```python
from build123d import *

# Parameters (mm, degrees)
F0_R     = 7
F0_R_2   = 2.25
F1_DEPTH = 2
F2_SIZE  = 1.99999


# Not quite as in the source:
# - a fillet or chamfer is up to 0.001 mm smaller than in the source, because OpenCascade refuses the exact size


with BuildPart() as f1:
    # F0 (on Top) → F1 (new body)
    with BuildSketch(Plane.XY):
        with BuildLine():
            ThreePointArc((11.7645575334, 8.4761539653), (10.9717281133, 9.333063578), (10.2530483272, 10.2530483272))
            ThreePointArc((10.2530483272, 10.2530483272), (0, 14.5), (-10.2530483272, 10.2530483272))
            ThreePointArc((-10.2530483272, 10.2530483272), (-10.9717281133, 9.333063578), (-11.7645575334, 8.4761539653))
            ThreePointArc((-11.7645575334, 8.4761539653), (-14.5, 0), (-11.7645575334, -8.4761539653))
            ThreePointArc((-11.7645575334, -8.4761539653), (-10.9717281133, -9.333063578), (-10.2530483272, -10.2530483272))
            ThreePointArc((-10.2530483272, -10.2530483272), (0, -14.5), (10.2530483272, -10.2530483272))
            ThreePointArc((10.2530483272, -10.2530483272), (10.9717281133, -9.333063578), (11.7645575334, -8.4761539653))
            ThreePointArc((11.7645575334, -8.4761539653), (13.7992044016, -4.4533086445), (14.5, 0))
            ThreePointArc((14.5, 0), (13.7992044016, 4.4533086445), (11.7645575334, 8.4761539653))
        make_face()
        Circle(F0_R, mode=Mode.SUBTRACT)
        with BuildLine():
            ThreePointArc((11.7645575334, 8.4761539653), (11.0445950741, 9.3950476129), (10.2530483272, 10.2530483272))
            ThreePointArc((10.2530483272, 10.2530483272), (10.9717281133, 9.333063578), (11.7645575334, 8.4761539653))
        make_face()
        with BuildLine():
            ThreePointArc((-11.7645575334, 8.4761539653), (-10.9717281133, 9.333063578), (-10.2530483272, 10.2530483272))
            ThreePointArc((-10.2530483272, 10.2530483272), (-11.0445950741, 9.3950476129), (-11.7645575334, 8.4761539653))
        make_face()
        with BuildLine():
            ThreePointArc((20, 4.5), (15.5484628484, 5.7966747348), (11.7645575334, 8.4761539653))
            ThreePointArc((11.7645575334, 8.4761539653), (13.7992044016, 4.4533086445), (14.5, 0))
            ThreePointArc((14.5, 0), (13.7992044016, -4.4533086445), (11.7645575334, -8.4761539653))
            ThreePointArc((11.7645575334, -8.4761539653), (15.5484628484, -5.7966747348), (20, -4.5))
            ThreePointArc((20, -4.5), (24.5, 0), (20, 4.5))
        make_face()
        with Locations((20, 0)):
            Circle(F0_R_2, mode=Mode.SUBTRACT)
        with BuildLine():
            ThreePointArc((-11.7645575334, -8.4761539653), (-14.5, 0), (-11.7645575334, 8.4761539653))
            ThreePointArc((-11.7645575334, 8.4761539653), (-15.5484628484, 5.7966747348), (-20, 4.5))
            ThreePointArc((-20, 4.5), (-24.5, 0), (-20, -4.5))
            ThreePointArc((-20, -4.5), (-15.5484628484, -5.7966747348), (-11.7645575334, -8.4761539653))
        make_face()
        with Locations((-20, 0)):
            Circle(F0_R_2, mode=Mode.SUBTRACT)
        with BuildLine():
            ThreePointArc((-10.2530483272, -10.2530483272), (-10.9717281133, -9.333063578), (-11.7645575334, -8.4761539653))
            ThreePointArc((-11.7645575334, -8.4761539653), (-11.0445950741, -9.3950476129), (-10.2530483272, -10.2530483272))
        make_face()
        with BuildLine():
            ThreePointArc((10.2530483272, -10.2530483272), (11.0445950741, -9.3950476129), (11.7645575334, -8.4761539653))
            ThreePointArc((11.7645575334, -8.4761539653), (10.9717281133, -9.333063578), (10.2530483272, -10.2530483272))
        make_face()
    extrude(amount=F1_DEPTH)

    # F2 (size 2 in the source; OpenCascade refuses exactly that, so slightly less here)
    f2_edges = [f1.edges().sort_by_distance(p)[0] for p in [
        (-7, 0, 2),
    ]]
    chamfer(f2_edges, length=F2_SIZE)


solid = f1.part
```
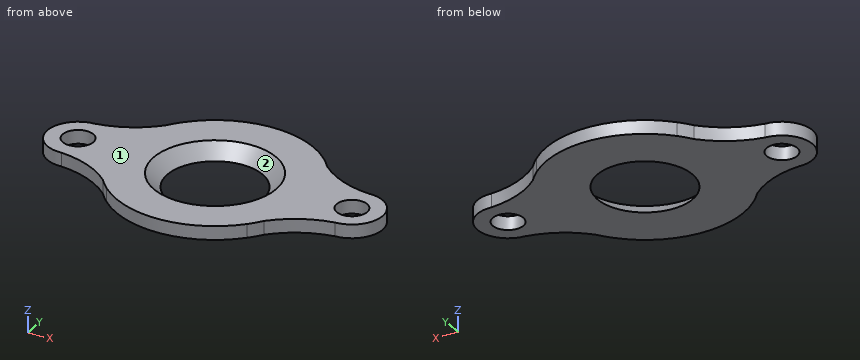
Could you check a few things on this model? Use its own coordinates, in mm. Face numbers are marked on the shaded views. Coordinates: 2 decimals unless noted, no trailing zeros. Loops run counter-clockwise (first coordinate to the right, second up) from the corner with the lowest first, then second, coordinate; pieces in that order, holes last. Notation, with made-up numbers: M -19,-17 L -7,-17 A16 cw -7,-6 Z; hole C 65,14 d10. An arc over 180 degrees is marked long. Put each result on its own line as item: value. Start each with the question number.
(1) Suppose I cut it at B-B on z = 1.1. Please give me the cut outline in (x, y), then the cut area to 3 significant figures.
(2) Thinking about a two-plate mould opening in X: for the marked faces 1 and 2, which applies, pulls with the +X half, pulls with the -X half, needs draft (parallel to the pull), parting line crosses it, or undercut?
(3) Suppose I cut it at D-D on x = 20.5. Please give me the cut outline in (y, z), then the cut area to 3 significant figures.
(4) Suppose I cut it at A-A on y = 0. Count the separate pieces of the cut face and the enclosed holes in it, then the cut area to 3 significant figures.
(5) I need wall thicknesses on line 1 (Y direction, x = 20, z = 1.3); line 2 (X direction, y = 0.25, z = 1.9); line 3 (X direction, y = 1, z = 1.85). Which ranges of each line are inside material? Lowest first, please. Write a range as from..to.
Solutions:
1. outline: M -20,-4.5 A14 cw -11.76,-8.48 A14.5 ccw 11.76,-8.48 A14 cw 20,-4.5 A4.5 ccw 20,4.5 A14 cw 11.76,8.48 A14.5 ccw -11.76,8.48 A14 cw -20,4.5 A4.5 ccw Z; hole C -20,0 d4.5; hole C 0,0 d16.2; hole C 20,0 d4.5
1. area: 618 mm2
2. face 1: needs draft
2. face 2: undercut
3. outline: M -4.47,0 L -2.19,0 L -2.19,2 L -4.47,2 Z; M 2.19,0 L 4.47,0 L 4.47,2 L 2.19,2 Z
3. area: 9.11 mm2
4. separate pieces: 4
4. enclosed holes: 0
4. area: 48.0 mm2
5. line 1: y = -4.5..-2.25, 2.25..4.5
5. line 2: x = -24.49..-22.24, -17.76..-8.9, 8.9..17.76, 22.24..24.49
5. line 3: x = -24.39..-22.02, -17.98..-8.79, 8.79..17.98, 22.02..24.39
